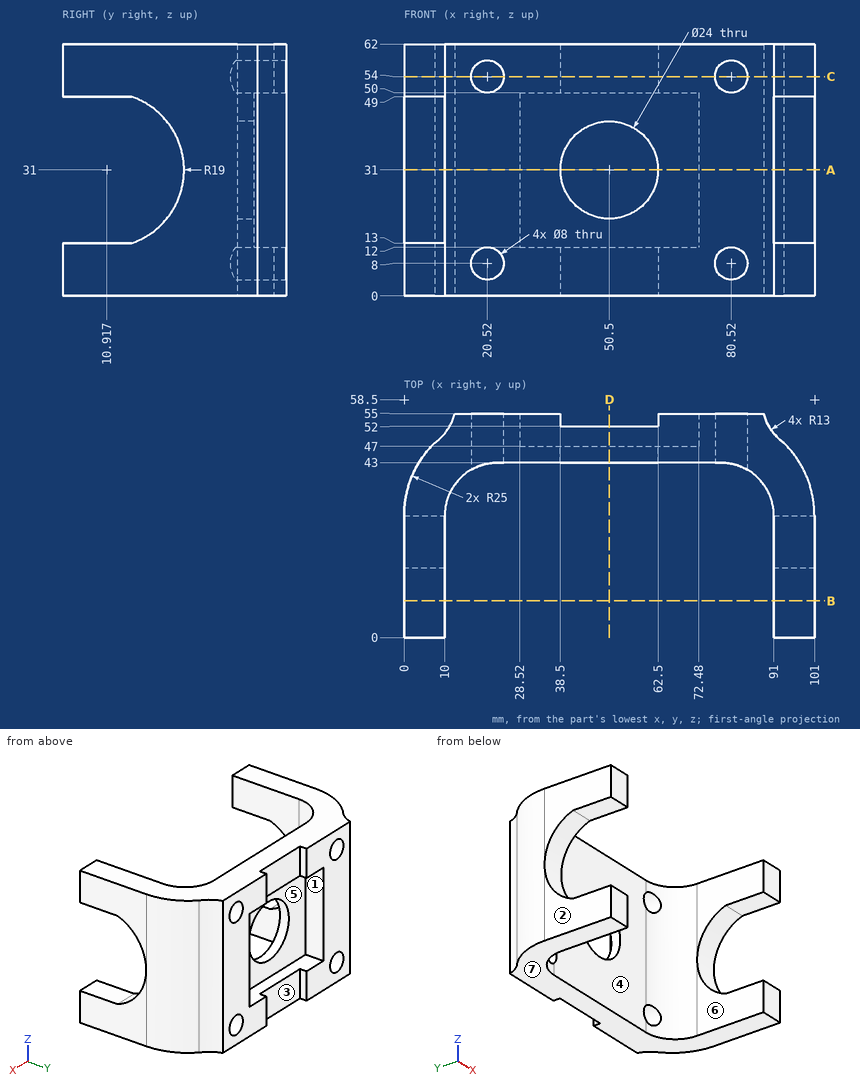
Input: dimensioned drawing with shaded views. Units: mm. Origin: part minimum x, y, z. A direction names the side the tool comes from. Round coordinates to 2 decimals unless told otherwise and drop trailing zeros. Write each loop counter-clockwise with the first axis right and the second up, starting at its lowest first coordinate (ties: lowest second). Pieces come first, ordered by that corner, then holes. Notation, with made-up numbers: (19.5, -3.75) -> (58.5, -3.75) arc R28 ccw to (58.5, 22.25) -> close; hole circle Ø7 at (-35, 18.25). An arc over 180 degrees is marked (long way). Use CSV: the item, a comma, the result in double quotes. Start each with the question number.
Q1. Section D-D (x = 50.5). Return loops of the section in (y, z).
Q2. Reachability of the marked faces 1, 2, 3 and 4 from +Z, -Z, +X, -X, +Y, -Y: full face, straight path, thin tool, end or side. Return the list, or none.
Q3. Line query: L1, parallel to Z at x = 4, y = 23; L2, parallel to X at y = 45.3, z = 31; L3, parallel to X at y = 40, z = 5.5. Output: solid intervals per line, ascending.
Q4. First-contact query: pin 1 Ø13 at (x, z) = (49, 8.5) entering from +Y; pin 2 Ø12 at (y, z) = (13, 39.5) entering from +X; pin 3 Ø2.5 at (y, z) = (52.5, 35.5) entering from -X; pin 4 Ø9 at (x, z) = (20.52, 54) entering from -Y. Flat tips, straight axial feed; report the tip coordinate or a pass-through.
Q5. Pull-direction query (Z, two-part tool) for the marked faces 5, 6 and 7; classes: pulls with the +Z half, pulls with the -Z half, needs draft (parallel to the pull), parting line crosses it, or undercut.
Q6. Section B-B (y = 9). Return loops of the section in (x, z).
Q7. Section A-A (z = 31). Return loops of the section in (x, y), plus the area to 3 significant figures.
Q8. Section C-C (z = 54). Return loops of the section in (x, y), plus the area to 3 significant figures.
Result sheet:
1,outline,"(43, 0) -> (52, 0) -> (52, 12) -> (47, 12) -> (47, 19) -> (43, 19) -> close; (43, 43) -> (47, 43) -> (47, 50) -> (52, 50) -> (52, 62) -> (43, 62) -> close"
2,face 1,"+Y"
2,face 2,"+Z, -Z, -X, +Y, -Y"
2,face 3,"+Z, -Z, +Y"
2,face 4,"+Z, -Z, -Y"
3,L1,"0 to 16.34, 45.66 to 62"
3,L2,"5.23 to 38.5, 62.5 to 95.77"
3,L3,"2.09 to 14.69, 86.31 to 98.91"
4,pin 1,"y = 52"
4,pin 2,"through"
4,pin 3,"x = 10.79"
4,pin 4,"y = 40.97"
5,face 5,"undercut"
5,face 6,"needs draft"
5,face 7,"pulls with the -Z half"
6,outline,"(0, 0) -> (10, 0) -> (10, 13) -> (0, 13) -> close; (0, 49) -> (10, 49) -> (10, 62) -> (0, 62) -> close; (91, 0) -> (101, 0) -> (101, 13) -> (91, 13) -> close; (91, 49) -> (101, 49) -> (101, 62) -> (91, 62) -> close"
7,outline,"(0, 29.92) -> (10, 29.92) -> (10, 30) arc R13 cw to (23, 43) -> (38.5, 43) -> (38.5, 47) -> (28.52, 47) -> (28.52, 55) -> (12.52, 55) arc R13 cw to (7.61, 47.96) arc R25 ccw to (0, 30) -> close; (62.5, 43) -> (78, 43) arc R13 cw to (91, 30) -> (91, 29.92) -> (101, 29.92) -> (101, 30) arc R25 ccw to (93.39, 47.96) arc R13 cw to (88.48, 55) -> (72.48, 55) -> (72.48, 47) -> (62.5, 47) -> close"
7,area,"864 mm²"
8,outline,"(0, 0) -> (10, 0) -> (10, 30) arc R13 cw to (16.52, 41.27) -> (16.52, 55) -> (12.52, 55) arc R13 cw to (7.61, 47.96) arc R25 ccw to (0, 30) -> close; (24.52, 43) -> (76.52, 43) -> (76.52, 55) -> (62.5, 55) -> (62.5, 52) -> (38.5, 52) -> (38.5, 55) -> (24.52, 55) -> close; (84.52, 41.25) arc R13 cw to (91, 30) -> (91, 0) -> (101, 0) -> (101, 30) arc R25 ccw to (93.39, 47.96) arc R13 cw to (88.48, 55) -> (84.52, 55) -> close"
8,area,"1,640 mm²"
